Part model, mm, in its own coordinate system. Face numbers are marked on the shaded views. Give positions to 0.01 mm unless a question says otherwise; leave off trailing zeros. Write each loop counter-clockwise with the first axis right and the second up, starting at its lowest first coordinate (ties: lowest second). Pieces come first, ordered by that corner, then holes. Notation, with made-up numbers: M 23,39.25 L 38,39.25 A24 cw 38,50.25 Z; hole C 52,4 d2. An arc over 180 degrees is marked long. Use a Markdown table: item, result.
```python
from build123d import *

# Parameters (mm, degrees)
SKETCH1_W            = 216
SKETCH1_H            = 127
BOSS_EXTRUDE1_DEPTH  = 10
FILLET1_R            = 10
FILLET2_R            = 10
SKETCH9_R            = 11.35
CUT_EXTRUDE4_DEPTH   = 7
SKETCH12_R           = 4.15
CUT_EXTRUDE5_DEPTH   = 7
SKETCH9_4_W          = 43
SKETCH9_4_H          = 43
CUT_EXTRUDE6_DEPTH   = 126.683133315
SKETCH13_W           = 43
SKETCH13_H           = 4
BOSS_EXTRUDE2_DEPTH  = 17
FILLET4_R            = 2
SKETCH17_W           = 43
SKETCH17_H           = 4
BOSS_EXTRUDE5_DEPTH  = 9
SKETCH18_W           = 43
SKETCH18_H           = 4
BOSS_EXTRUDE6_DEPTH  = 17
SKETCH19_W           = 43
SKETCH19_H           = 4
BOSS_EXTRUDE7_DEPTH  = 9
FILLET5_R            = 2
SKETCH20_R           = 1.85
CUT_EXTRUDE7_DEPTH   = 9
SKETCH23_R           = 1.85
CUT_EXTRUDE8_DEPTH   = 9
SKETCH25_R           = 15
BOSS_EXTRUDE9_DEPTH  = 40
SKETCH26_R           = 4.15
BOSS_EXTRUDE10_DEPTH = 15
SKETCH27_R           = 4.15
BOSS_EXTRUDE11_DEPTH = 15
FILLET9_R            = 2
FILLET10_R           = 2
SKETCH28_R           = 7.5
CUT_EXTRUDE9_DEPTH   = 142.142658328


with BuildPart() as part:
    # Sketch1 → Boss-Extrude1 (new body)
    with BuildSketch(Plane.XY):
        Rectangle(SKETCH1_W, SKETCH1_H)
    extrude(amount=BOSS_EXTRUDE1_DEPTH)

    # Fillet1
    fillet1_edges = [part.edges().sort_by_distance(p)[0] for p in [
        (-108, 63.5, 5),
    ]]
    fillet(fillet1_edges, radius=FILLET1_R)

    # Fillet2
    fillet2_edges = [part.edges().sort_by_distance(p)[0] for p in [
        (108, -63.5, 5),
        (-108, -63.5, 5),
        (108, 63.5, 5),
    ]]
    fillet(fillet2_edges, radius=FILLET2_R)

    # Sketch9 → Cut-Extrude4 (cut)
    with BuildSketch(Plane(origin=(0, 0, 0), x_dir=(-1, 0, 0), z_dir=(0, 0, -1))):
        with Locations((-4, 0)):
            Circle(SKETCH9_R)
    extrude(amount=-CUT_EXTRUDE4_DEPTH, mode=Mode.SUBTRACT)

    # Sketch12 → Cut-Extrude5 (cut)
    with BuildSketch(Plane(origin=(0, 0, 7), x_dir=(-1, 0, 0), z_dir=(0, 0, -1))):
        with Locations((-4, 0)):
            Circle(SKETCH12_R)
    extrude(amount=-CUT_EXTRUDE5_DEPTH, mode=Mode.SUBTRACT)

    # Sketch9_4 → Cut-Extrude6 (cut, through all)
    with BuildSketch(Plane(origin=(0, 0, 0), x_dir=(-1, 0, 0), z_dir=(0, 0, -1))):
        with Locations((-59, 0)):
            Rectangle(SKETCH9_4_W, SKETCH9_4_H)
    extrude(amount=-CUT_EXTRUDE6_DEPTH, mode=Mode.SUBTRACT)

    # Sketch13 → Boss-Extrude2 (add)
    with BuildSketch(Plane(origin=(0, 0, 0), x_dir=(-1, 0, 0), z_dir=(0, 0, -1))):
        with Locations((-59, -23.5)):
            Rectangle(SKETCH13_W, SKETCH13_H)
    extrude(amount=BOSS_EXTRUDE2_DEPTH)

    # Fillet4
    fillet4_edges = [part.edges().sort_by_distance(p)[0] for p in [
        (37.5, -23.5, 0),
        (80.5, -23.5, 0),
        (59, -25.5, 0),
    ]]
    fillet(fillet4_edges, radius=FILLET4_R)

    # Sketch17 → Boss-Extrude5 (add)
    with BuildSketch(Plane(origin=(0, -21.5, 0), x_dir=(1, 0, 0), z_dir=(0, 1, 0))):
        with Locations((59, 15)):
            Rectangle(SKETCH17_W, SKETCH17_H)
    extrude(amount=BOSS_EXTRUDE5_DEPTH)

    # Sketch18 → Boss-Extrude6 (add)
    with BuildSketch(Plane(origin=(0, 0, 0), x_dir=(-1, 0, 0), z_dir=(0, 0, -1))):
        with Locations((-59, 23.5)):
            Rectangle(SKETCH18_W, SKETCH18_H)
    extrude(amount=BOSS_EXTRUDE6_DEPTH)

    # Sketch19 → Boss-Extrude7 (add)
    with BuildSketch(Plane(origin=(0, 21.5, 0), x_dir=(-1, 0, 0), z_dir=(0, -1, 0))):
        with Locations((-59, 15)):
            Rectangle(SKETCH19_W, SKETCH19_H)
    extrude(amount=BOSS_EXTRUDE7_DEPTH)

    # Fillet5
    fillet5_edges = [part.edges().sort_by_distance(p)[0] for p in [
        (37.5, 23.5, 0),
        (59, 25.5, 0),
        (80.5, 23.5, 0),
    ]]
    fillet(fillet5_edges, radius=FILLET5_R)

    # Sketch20 → Cut-Extrude7 (cut)
    with BuildSketch(Plane(origin=(0, 0, -17), x_dir=(-1, 0, 0), z_dir=(0, 0, -1))):
        with Locations((-43.15, -16)):
            Circle(SKETCH20_R)
        with Locations((-74.85, -16)):
            Circle(SKETCH20_R)
    extrude(amount=-CUT_EXTRUDE7_DEPTH, mode=Mode.SUBTRACT)

    # Sketch23 → Cut-Extrude8 (cut)
    with BuildSketch(Plane(origin=(0, 0, -17), x_dir=(-1, 0, 0), z_dir=(0, 0, -1))):
        with Locations((-43.15, 15.85)):
            Circle(SKETCH23_R)
        with Locations((-74.85, 16)):
            Circle(SKETCH23_R)
    extrude(amount=-CUT_EXTRUDE8_DEPTH, mode=Mode.SUBTRACT)

    # Sketch25 → Boss-Extrude9 (add)
    with BuildSketch(Plane(origin=(0, 0, 0), x_dir=(-1, 0, 0), z_dir=(0, 0, -1))):
        with Locations(Location((50.981638517, -43.5, 0), (0, 0, 180))):
            Circle(SKETCH25_R)
        with Locations(Location((50.981638517, 43.5, 0), (0, 0, 180))):
            Circle(SKETCH25_R)
    extrude(amount=BOSS_EXTRUDE9_DEPTH)

    # Sketch26 → Boss-Extrude10 (add)
    with BuildSketch(Plane(origin=(0, 0, -40), x_dir=(-1, 0, 0), z_dir=(0, 0, -1))):
        with Locations((50.981638517, -43.5)):
            Circle(SKETCH26_R)
    extrude(amount=BOSS_EXTRUDE10_DEPTH)

    # Sketch27 → Boss-Extrude11 (add)
    with BuildSketch(Plane(origin=(0, 0, -40), x_dir=(-1, 0, 0), z_dir=(0, 0, -1))):
        with Locations((50.981638517, 43.5)):
            Circle(SKETCH27_R)
    extrude(amount=BOSS_EXTRUDE11_DEPTH)

    # Fillet9
    fillet9_edges = [part.edges().sort_by_distance(p)[0] for p in [
        (-65.981638517, -43.5, 0),
    ]]
    fillet(fillet9_edges, radius=FILLET9_R)

    # Fillet10
    fillet10_edges = [part.edges().sort_by_distance(p)[0] for p in [
        (-65.981638517, 43.5, 0),
    ]]
    fillet(fillet10_edges, radius=FILLET10_R)

    # Sketch28 → Cut-Extrude9 (cut, through all)
    with BuildSketch(Plane.XY.offset(10)):
        with Locations((-84.811667967, 46.37)):
            Circle(SKETCH28_R)
        with Locations((-84.811667967, -46.37)):
            Circle(SKETCH28_R)
        with Locations((95.674047271, -46.369786546)):
            Circle(SKETCH28_R)
        with Locations((93.399057455, 46.37)):
            Circle(SKETCH28_R)
    extrude(amount=-CUT_EXTRUDE9_DEPTH, mode=Mode.SUBTRACT)


solid = part.part
```
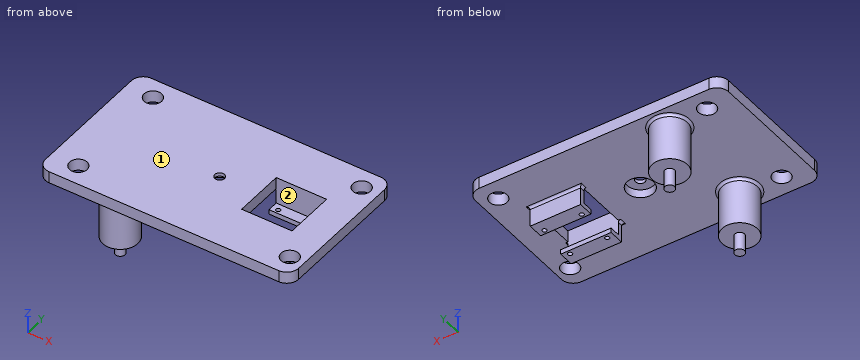
1. Drill centre lines: L1, parallel to Y at x = 74.85, z = -15.6; L2, parallel to X at y = 46, z = 4; L3, parallel to Y at x = 38.5, z = -8. Where is each one in solid material? Low to high.
Findings below:
| item | result |
|---|---|
| L1 | -25.5 to -17.85, -14.15 to -12.5, 12.5 to 14.15, 17.85 to 25.5 |
| L2 | -108 to -92.3, -77.32 to 85.91, 100.89 to 108 |
| L3 | -25.5 to -21.5, 21.5 to 25.5 |
2. Two-plate mould, pull along Y, no slides. Class the marked faces 1 and 2: released by +Y, released by -Y, zero draft, split by the parting line, or undercut.
Findings below:
| item | result |
|---|---|
| face 1 | zero draft |
| face 2 | undercut |
3. Cut at D-D, the plane x = -15. Give the cut face in (y, z), then the cut area to 3 significant figures.
Findings below:
| item | result |
|---|---|
| outline | M -63.5,0 L 63.5,0 L 63.5,10 L -63.5,10 Z |
| area | 1,270 mm2 |
4. Drop flat-ended pins along their axis: P1, Ø1, axis at x = -54, y = -37.5, coming from the -Z side; P2, Ø3, axis at x = 43.15, y = 15.85, coming from the +Z side; P3, Ø6.5, axis at x = 67.5, y = -21, coming from the -Z side; P4, Ø24, axis at x = -52, y = 36.5, coming from the -Z side. Give the stop position or say it passes through.
Findings below:
| item | result |
|---|---|
| P1 | z = -40 |
| P2 | through |
| P3 | z = -17 |
| P4 | z = -55 |
5. Cut at B-B, the plane z = -36. Give the cut face in (x, y), then the cut area to 3 significant figures.
Findings below:
| item | result |
|---|---|
| outline | C -50.98,-43.5 d30; C -50.98,43.5 d30 |
| area | 1,410 mm2 |
6. Cut at A-A, the plane y = 0. Give the cut face in (x, z).
Findings below:
| item | result |
|---|---|
| outline | M -108,0 L -7.35,0 L -7.35,7 L -0.15,7 L -0.15,10 L -108,10 Z; M 8.15,7 L 15.35,7 L 15.35,0 L 37.5,0 L 37.5,10 L 8.15,10 Z; M 80.5,0 L 108,0 L 108,10 L 80.5,10 Z |
7. Cut at C-C, the plane x = -86. Give the cut face in (y, z).
Findings below:
| item | result |
|---|---|
| outline | M -63.5,0 L -53.78,0 L -53.78,10 L -63.5,10 Z; M -38.96,0 L 38.96,0 L 38.96,10 L -38.96,10 Z; M 53.78,0 L 63.5,0 L 63.5,10 L 53.78,10 Z |
